Input: part model. Units: mm. Frame: model coordinates. A direction names the side the tool comes from. Give positions to 0.01 mm unless a question says otherwise; leave off trailing zeros. Loops run counter-clockwise (first coordinate to the right, second up) from the corner with the lowest first, then second, coordinate; pieces in that order, holes last. Notation, with made-up numbers: M 53,-34.5 L 109,-34.5 A23 ccw 109,4.5 Z; hole C 15.5,0 d2. An arc over 180 degrees is marked long. One line per item, written item: value. Start each with the question number.
(1) Section D-D on x = -9. Output: boundary loops of the cut face in (y, z).
(2) Section C-C on z = -55. Output: boundary loops of the cut face in (x, y).
(3) Pull-direction query (Y, two-part tool) for faces 3 (the flat face through (0, 0, 100)), 4 (the cylindrical face through (20.03, -6.31, 97.46)), 5 (the cylindrical face through (-14.985, 0.66, 1.33)); classes: released by +Y, released by -Y, zero draft, split by the parting line, or undercut.
(4) Access query for faces 1 (the cylindrical face through (-2.934, 16.576, -54.885)), 2 (the cylindrical face through (-4.01, 18.06, -1.33)). Directions: +Z, -Z, +X, -X, +Y, -Y. A direction counts if a zero-diameter tool reaches every point of the face in a straight line with its end or side. Return the directions, or none.
(5) Ray query, line 1 along Y through (x, z) = (0, -28); line 2 along Z through (x, y) = (0, -17); line 3 along Y through (x, z) = (3, -63). Return the intervals inside material, ascending. Write a range as from..to.
(6) Section A-A on x = 0. Output: boundary loops of the cut face in (y, z).
(7) Pin query (flat end, axial travel): P1, Ø1, axis at x = 15, y = -14, coming from the -Z side; P2, Ø9.5, axis at x = 0, z = -54.5, coming from the +Y side; P3, Ø6, axis at x = 12, z = -52, coming from the -Y side. Return the tip coordinate at first contact, or that it passes through.
(8) Section B-B on y = 0. Output: boundary loops of the cut face in (x, z), plus the area to 3 significant figures.
Autodesk Inventor part; units mm, degrees
ref_plane "Work Plane4" through (0, 18.5, 0) normal (0, 1, 0) x (-1, 0, 0)
ref_plane "YZ Plane" through (0, 0, 0) normal (1, 0, 0) x (0, 1, 0)
ref_plane "XZ Plane" through (0, 0, 0) normal (0, 1, 0) x (-1, 0, 0)
sketch "Sketch1" plane through (0, 0, 0) normal (0, 0, 1) x (1, 0, 0)
  circle A0 centre (0, 0) radius 18.5
  circle A1 centre (0, 0) radius 15
  dimension "d0" = 37
  dimension "d1" = 30
extrude "Extrusion1" add sketch "Sketch1" along normal mid plane 190
ref_plane "Work Plane4" through (0, 18.5, 0) normal (0, 1, 0) x (-1, 0, 0)
sketch "Sketch4" plane through (0, 18.5, 0) normal (0, 1, 0) x (-1, 0, 0)
  line L0 (-18.5, -95) -> (18.5, -95)
  line L1 (18.5, -95) -> (18.5, 95)
  line L2 (-18.5, -95) -> (18.5, -95)
  line L3 (18.5, 95) -> (-18.5, 95)
  point P0 (0, 0)
  point P1 (0, -54.5)
  dimension "d14" = 40.5
  dimension "d22" = 190
  dimension "d23" = 18.5
hole "Hole1" at (0, 18.5, -54.5) direction (0, -1, 0) diameter 5.9175 depth 19.1 tip angle 118
mirror "Mirror2" about plane through (0, 0, 0) normal (0, 1, 0) of "Hole1"
sketch "Sketch5" plane through (0, 0, 95) normal (0, 0, 1) x (1, 0, 0)
  circle A0 centre (0, 0) radius 21
  dimension "d24" = 42
extrude "Extrusion3" add sketch "Sketch5" along normal blind 5
properties part number "EjeRodilla"
Output values:
1. outline: M -18.97,95 L -16.16,95 L -16.16,-95 L -12,-95 L -12,95 L 12,95 L 12,-95 L 16.16,-95 L 16.16,95 L 18.97,95 L 18.97,100 L -18.97,100 Z
2. outline: M -2.92,-18.27 L -2.92,-14.71 A15 cw -2.92,14.71 L -2.92,18.27 A18.5 ccw Z; M 2.92,-18.27 A18.5 ccw 2.92,18.27 L 2.92,14.71 A15 cw 2.92,-14.71 Z
3. face 3: zero draft
3. face 4: split by the parting line
3. face 5: undercut
4. face 1: +Y, -Y
4. face 2: -Z
5. line 1: y = -18.5..-15, 15..18.5
5. line 2: z = -95..-57.46, -51.54..100
5. line 3: y = -18.26..-14.7, 14.7..18.26
6. outline: M -21,95 L -18.5,95 L -18.5,-51.54 L -15,-51.54 L -15,95 L 15,95 L 15,-51.54 L 18.5,-51.54 L 18.5,95 L 21,95 L 21,100 L -21,100 Z; M -18.5,-95 L -15,-95 L -15,-57.46 L -18.5,-57.46 Z; M 15,-95 L 18.5,-95 L 18.5,-57.46 L 15,-57.46 Z
7. P1: stops at z = 95
7. P2: stops at y = 18.5
7. P3: stops at y = -16.16
8. outline: M -21,95 L -18.5,95 L -18.5,-95 L -15,-95 L -15,95 L 15,95 L 15,-95 L 18.5,-95 L 18.5,95 L 21,95 L 21,100 L -21,100 Z
8. area: 1,540 mm²
